Answer from the drawing. Dimensions are ordinates in mm from the lowest x, y and z of the part. A direction names the side the tool comes from. Round coordinates to 2 decimals unless told otherwise and drop trailing zeros. Write each loop counter-clockwise with the first axis right and the second up, starting at its lowest first coordinate (ties: lowest second). Pieces come first, ordered by that corner, then holes. Notation, with made-up numbers: M 55,71 L 105,71 A13 ccw 105,91 Z; hole C 27.5,36.25 d9. An arc over 180 degrees is marked long. One line per item, written item: value. Start each with the question number.
(1) Given P1, Ø1, axis at x = 11, y = 30.5, coming from the -Z side, flat-ended and moving along its own axis, determine where the tip first touches the part or whether it passes through.
(2) Section C-C (z = 40) is taken. Determine the outline of the cut face in (x, y) (1 decimal).
(3) Consider probe 1 along Y at (x, z) = (35, 32) (1 decimal); probe 2 along X at (y, z) = (14.5, 10); probe 3 along Z at (x, y) = (7, 3). Determine where each line is inside the solid, lowest interval first.
(4) Section B-B (y = 21) is taken. Determine the outline of the cut face in (x, z).
(5) For a pull along X with two mould halves and no side action, classify the marked faces 3, 4, 5 and 6 as released by +X, released by -X, zero draft, split by the parting line, or undercut.
(6) Section A-A (x = 7) is taken. Determine the outline of the cut face in (y, z) (1 decimal).
(7) For the marked faces 1 and 2, determine the directions among +Z, -Z, +X, -X, +Y, -Y from which every point of the face is accessible in a straight line to the end or side of a thin tool.
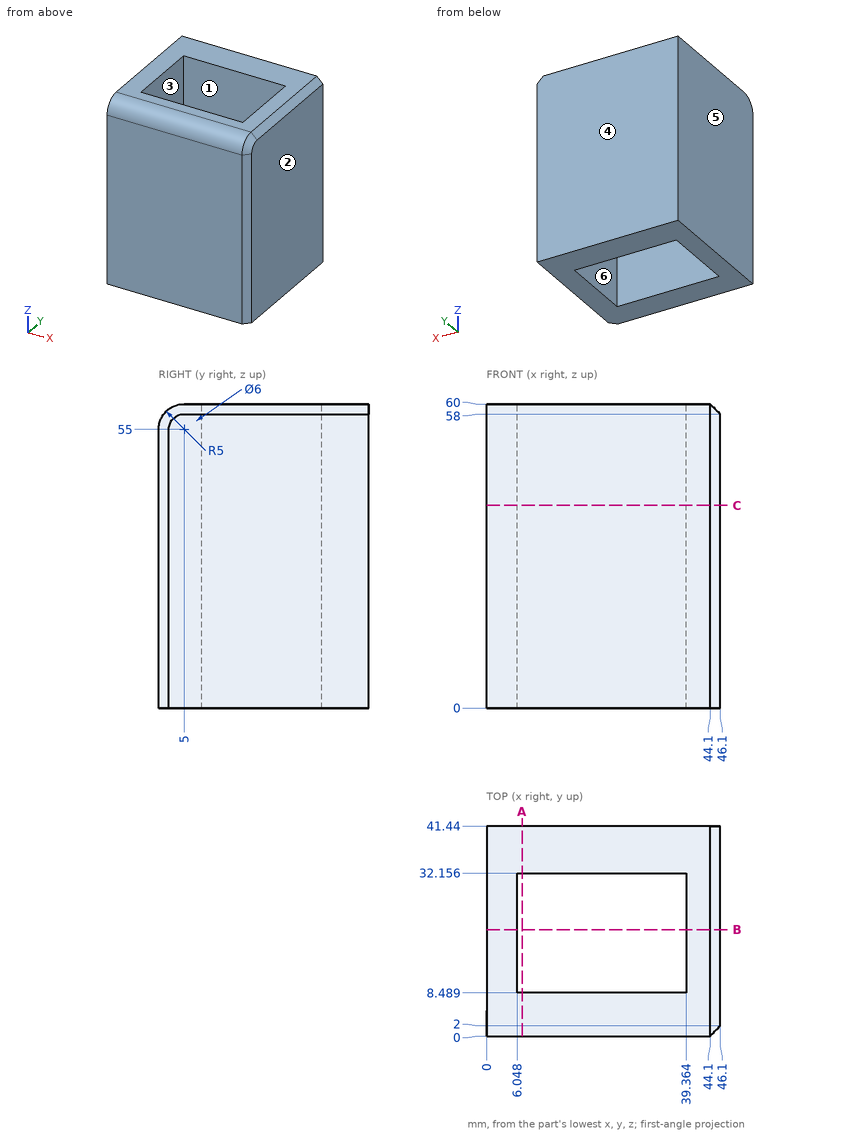
Recorded:
1. P1: passes through
2. outline: M 0,0 L 44.1,0 L 46.1,2 L 46.1,41.4 L 0,41.4 Z; hole M 6,8.5 L 39.4,8.5 L 39.4,32.2 L 6,32.2 Z
3. probe 1: y = 0 to 8.5, 32.2 to 41.4
3. probe 2: x = 0 to 6.05, 39.36 to 46.1
3. probe 3: z = 0 to 59.58
4. outline: M 0,0 L 6.05,0 L 6.05,60 L 0,60 Z; M 39.36,0 L 46.1,0 L 46.1,58 L 44.1,60 L 39.36,60 Z
5. face 3: undercut
5. face 4: zero draft
5. face 5: released by -X
5. face 6: undercut
6. outline: M 0,0 L 8.5,0 L 8.5,60 L 5,60 A5 ccw 0,55 Z; M 32.2,0 L 41.4,0 L 41.4,60 L 32.2,60 Z
7. face 1: +Z, -Z
7. face 2: +Z, -Z, +X, +Y, -Y
